```python
from build123d import *

# Parameters (mm, degrees)
ESQUISSE1_R             = 13
BOSS_EXTRU_1_DEPTH      = 11.5
ESQUISSE2_R             = 2
ENL_V_MAT_EXTRU_1_DEPTH = 5
ESQUISSE3_R             = 3
ENL_V_MAT_EXTRU_2_DEPTH = 4.5


with BuildPart() as part:
    # Esquisse1 → Boss.-Extru.1 (new body)
    with BuildSketch(Plane.XY):
        Circle(ESQUISSE1_R)
    extrude(amount=BOSS_EXTRU_1_DEPTH)

    # Esquisse2 → Enlèv. mat.-Extru.1 (cut)
    with BuildSketch(Plane.XY.offset(11.5)):
        with Locations((0, 8.5)):
            Circle(ESQUISSE2_R)
        with Locations((-7.361215932, 4.25)):
            Circle(ESQUISSE2_R)
        with Locations((-7.361215932, -4.25)):
            Circle(ESQUISSE2_R)
        with Locations((0, -8.5)):
            Circle(ESQUISSE2_R)
        with Locations((7.361215932, -4.25)):
            Circle(ESQUISSE2_R)
        with Locations((7.361215932, 4.25)):
            Circle(ESQUISSE2_R)
    extrude(amount=-ENL_V_MAT_EXTRU_1_DEPTH, mode=Mode.SUBTRACT)

    # Esquisse3 → Enlèv. mat.-Extru.2 (cut)
    with BuildSketch(Plane.XY.offset(11.5)):
        Circle(ESQUISSE3_R)
    extrude(amount=-ENL_V_MAT_EXTRU_2_DEPTH, mode=Mode.SUBTRACT)


solid = part.part
```
The model under review builds one solid part; all positions refer to its coordinate system, in mm. A direction names the side the tool comes from. Give positions to 0.01 mm unless a question says otherwise; leave off trailing zeros. Write each loop counter-clockwise with the first axis right and the second up, starting at its lowest first coordinate (ties: lowest second). Pieces come first, ordered by that corner, then holes. Notation, with made-up numbers: M 16,62 L 60,62 A30 ccw 60,91 Z; hole C 45.25,76 d3. An arc over 180 degrees is marked long. Answer in a Markdown table with one row per item.
Item 1: For P1, Ø5, axis at y = 3, z = 3, coming from the +X side; P2, Ø1.5, axis at x = 1.5, z = 9.5, coming from the -Y side; P3, Ø3.5, axis at x = 0, y = 8.5, coming from the +Z side, all flat-tipped, find the tip position at first contact; note any pin that passes through.
Check sheet entries:
| item | result |
|---|---|
| P1 | x = 12.99 |
| P2 | y = -12.98 |
| P3 | z = 6.5 |
Item 2: Add section B-B on y = 0. Give the boundary of the cut face in (x, z).
Check sheet entries:
| item | result |
|---|---|
| outline | M -13,0 L 13,0 L 13,11.5 L 3,11.5 L 3,7 L -3,7 L -3,11.5 L -13,11.5 Z |
Item 3: Add section C-C on x = 0. Give the boundary of the cut face in (y, z), plus the area to 3 significant figures.
Check sheet entries:
| item | result |
|---|---|
| outline | M -13,0 L 13,0 L 13,11.5 L 10.5,11.5 L 10.5,6.5 L 6.5,6.5 L 6.5,11.5 L 3,11.5 L 3,7 L -3,7 L -3,11.5 L -6.5,11.5 L -6.5,6.5 L -10.5,6.5 L -10.5,11.5 L -13,11.5 Z |
| area | 232 mm2 |
Item 4: Add section A-A on z = 8. Give the boundary of the cut face in (x, y).
Check sheet entries:
| item | result |
|---|---|
| outline | C 0,0 d26; hole C -7.36,-4.25 d4; hole C -7.36,4.25 d4; hole C 0,0 d6; hole C 0,-8.5 d4; hole C 0,8.5 d4; hole C 7.36,-4.25 d4; hole C 7.36,4.25 d4 |
Item 5: Tool access review of faces 1 (the face through (0, 0, 0)), 2 (the face through (-7, 4, 6.5)): name each direction out of +Z, -Z, +X, -X, +Y, -Y from which nothing blocks a thin tool from reaching the whole face with its end or side.
Check sheet entries:
| item | result |
|---|---|
| face 1 | -Z, +X, -X, +Y, -Y |
| face 2 | +Z |
Item 6: Draft analysis for pull direction X (two halves, no side actions). For faces 3 (the face through (-10.316, -7.91, 5.67)), 4 (the face through (3, -3, 11.5)), 5 (the face through (-5.514, -5.016, 9.035)), state which applies: +X half, -X half, draft (parallel to the pull), parting line (faces both ways), or undercut.
Check sheet entries:
| item | result |
|---|---|
| face 3 | parting line |
| face 4 | draft |
| face 5 | undercut |
Item 7: For line 1 along Y through (x, z) = (0, 8.7); line 2 along Y through (x, z) = (-6.75, 7.75); line 3 along Y through (x, z) = (-1.25, 7.5), list the stretches that pass through material, from the lowest coordinate up.
Check sheet entries:
| item | result |
|---|---|
| line 1 | -13 to -10.5, -6.5 to -3, 3 to 6.5, 10.5 to 13 |
| line 2 | -11.11 to -6.15, -2.35 to 2.35, 6.15 to 11.11 |
| line 3 | -12.94 to -10.06, -6.94 to -2.73, 2.73 to 6.94, 10.06 to 12.94 |
Item 8: Add section D-D on z = 3.25. Give the boundary of the cut face in (x, y).
Check sheet entries:
| item | result |
|---|---|
| outline | C 0,0 d26 |
